from build123d import *

# Parameters (mm, degrees)
F1_DEPTH  = 16
F3_DEPTH  = 25
F4_SIZE   = 1
F11_ANGLE = 180
F14_DEPTH = 2
F16_DEPTH = 2


with BuildPart() as f1:
    # F0 (on Right) → F1 (new body)
    with BuildSketch(Plane.YZ):
        with BuildLine():
            Line((0, 7), (0, 0))
            Line((0, 0), (150, 0))
            Line((150, 0), (150, 7))
            ThreePointArc((150, 7), (148.5355339059, 10.5355339059), (145, 12))
            Line((145, 12), (128.050036002, 10.517070303))
            Line((128.050036002, 10.517070303), (127.1432693018, 20.8814611121))
            Line((127.1432693018, 20.8814611121), (113.1965435286, 19.6612807136))
            Line((113.1965435286, 19.6612807136), (113.8937894705, 11.6917231289))
            Line((113.8937894705, 11.6917231289), (5.5800139851, 2.2154956702))
            Line((5.5800139851, 2.2154956702), (4.9427024368, 9.5))
            Line((4.9427024368, 9.5), (20, 9.5))
            Line((20, 9.5), (20, 12))
            Line((20, 12), (5, 12))
            ThreePointArc((5, 12), (1.4644660941, 10.5355339059), (0, 7))
        make_face()
    extrude(amount=F1_DEPTH)

    # F2 (on face) → F3 (cut)
    with BuildSketch(Plane(origin=(0, 114.0437613881, 9.9775362673), x_dir=(1, 0, 0), z_dir=(0, -0.9961946981, -0.0871557427))):
        with BuildLine():
            Line((6, 9.7207347769), (6, 6.8026639789))
            ThreePointArc((6, 6.8026639789), (8, 2.6707347769), (10, 6.8026639789))
            Line((10, 6.8026639789), (10, 9.7207347769))
            Line((10, 9.7207347769), (11.5, 9.7207347769))
            ThreePointArc((11.5, 9.7207347769), (12.2071067812, 9.4278415581), (12.5, 8.7207347769))
            Line((12.5, 8.7207347769), (12.5, 4.7207347769))
            ThreePointArc((12.5, 4.7207347769), (13.3786796564, 2.5994144334), (15.5, 1.7207347769))
            Line((15.5, 1.7207347769), (18.5, 1.7207347769))
            Line((18.5, 1.7207347769), (18.5, 10.7207347769))
            Line((18.5, 10.7207347769), (-2.5, 10.7207347769))
            Line((-2.5, 10.7207347769), (-2.5, 1.7207347769))
            Line((-2.5, 1.7207347769), (0.5, 1.7207347769))
            ThreePointArc((0.5, 1.7207347769), (2.6213203436, 2.5994144334), (3.5, 4.7207347769))
            Line((3.5, 4.7207347769), (3.5, 8.7207347769))
            ThreePointArc((3.5, 8.7207347769), (3.7928932188, 9.4278415581), (4.5, 9.7207347769))
            Line((4.5, 9.7207347769), (6, 9.7207347769))
        make_face()
    extrude(amount=-F3_DEPTH, mode=Mode.SUBTRACT)

    # F4
    f4_edges = [f1.edges().sort_by_distance(p)[0] for p in [
        (6, 120.169906, 20.271371),
        (10, 120.169906, 20.271371),
    ]]
    chamfer(f4_edges, length=F4_SIZE)


with BuildPart() as f5_1:
    # F5: copy of F1
    add(f1.part.moved(Location((30, 0, 0))))


with BuildPart() as f6_1:
    # F6: copy of F5_1
    add(f5_1.part.moved(Location((30, 0, 0))))


with BuildPart() as f7_1:
    # F7: copy of F1
    add(f1.part.moved(Location((0, 160, 0))))


with BuildPart() as f8_1:
    # F8: copy of F5_1
    add(f5_1.part.moved(Location((0, 160, 0))))


with BuildPart() as f9_1:
    # F9: copy of F6_1
    add(f6_1.part.moved(Location((0, 160, 0))))


with BuildPart() as f8_1_1:
    # F11: moved
    add(f8_1.part.rotate(Axis((0, 0, 25), (0, 0, 1)), F11_ANGLE))


with BuildPart() as f9_1_1:
    # F11: moved
    add(f9_1.part.rotate(Axis((0, 0, 25), (0, 0, 1)), F11_ANGLE))


with BuildPart() as f7_1_1:
    # F11: moved
    add(f7_1.part.rotate(Axis((0, 0, 25), (0, 0, 1)), F11_ANGLE))


with BuildPart() as f7_1_2:
    # F12: moved
    add(f7_1_1.part.moved(Location((91, 310, 0))))

    # F13 (on face) → F14 (join)
    with BuildSketch(Plane.YZ.offset(91)):
        with BuildLine():
            Line((0, 7), (0, 0))
            Line((0, 0), (150, 0))
            Line((150, 0), (150, 7))
            ThreePointArc((150, 7), (148.5355339059, 10.5355339059), (145, 12))
            Line((145, 12), (5, 12))
            ThreePointArc((5, 12), (1.4644660941, 10.5355339059), (0, 7))
        make_face()
    extrude(amount=F14_DEPTH)


with BuildPart() as f8_1_2:
    # F12: moved
    add(f8_1_1.part.moved(Location((91, 310, 0))))


with BuildPart() as f9_1_2:
    # F12: moved
    add(f9_1_1.part.moved(Location((91, 310, 0))))


with BuildPart() as f1_1:
    add(f1.part)

    add(f5_1.part)  # F16 merges F5_1

    add(f6_1.part)  # F16 merges F6_1

    add(f7_1_2.part)  # F16 merges F7_1

    add(f8_1_2.part)  # F16 merges F8_1

    add(f9_1_2.part)  # F16 merges F9_1
    # F15 (on face) → F16 (join)
    with BuildSketch(Plane(origin=(0, 0, 0), x_dir=(0, -1, 0), z_dir=(-1, 0, 0))):
        with BuildLine():
            Line((-150, 0), (0, 0))
            Line((0, 0), (0, 7))
            ThreePointArc((0, 7), (-1.4644660941, 10.5355339059), (-5, 12))
            Line((-5, 12), (-145, 12))
            ThreePointArc((-145, 12), (-148.5355339059, 10.5355339059), (-150, 7))
            Line((-150, 7), (-150, 0))
        make_face()
    extrude(amount=F16_DEPTH)


solid = f1_1.part
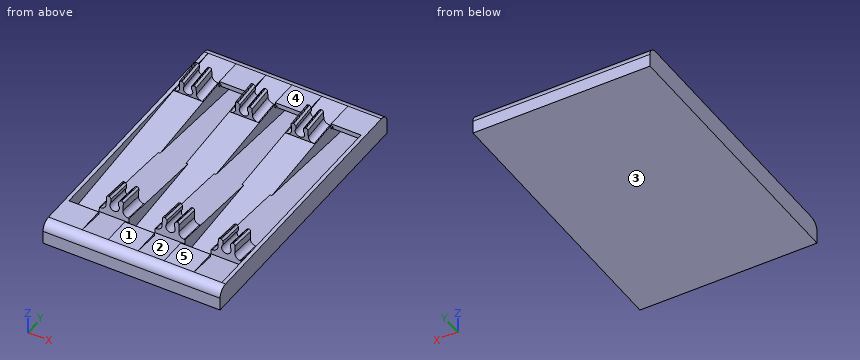
Source: CAD feature listing. Evaluate the final solid. Frame: model axes, mm. Face numbers are marked on the shaded views. A direction names the side the tool comes from. Give positions to 0.01 mm unless a question says otherwise; leave off trailing zeros. Order: outer loops, then holes, each group sorted by start corner. A loop starts at its lowest first (then second) coordinate and runs counter-clockwise, first axis right, second up. Notation, with made-up numbers: (83, 55) -> (136, 55) arc R24 ccw to (136, 75) -> close; hole circle Ø8 at (2, 39.25). An arc over 180 degrees is marked (long way). Write item = value, one per line.
Q1. Set-up query: the marked faces 3, 4 and 5. Return all of +Z, -Z, +X, -X, +Y, -Y with unobstructed straight access to the full face (end or side cutting, diameter ignored); none if empty.
Data:
face_3 = -Z, +X, -X, +Y, -Y
face_4 = +Z, +X, -X, +Y
face_5 = +Z, +X, -X, -Y
Q2. Pull-direction query (Y, two-part tool) for the marked faces 1 and 2; classes: released by +Y, released by -Y, zero draft, split by the parting line, or undercut.
Data:
face_1 = zero draft
face_2 = undercut
Q3. Cut plane D-D, the plane y = 17. Output: boundary loops of the cut face in (x, z), and give its area (3 significant figures).
Data:
outline = (-2, 0) -> (93, 0) -> (93, 12) -> (91, 12) -> (91, 10.95) -> (76, 10.95) -> (76, 12) -> (60, 12) -> (60, 10.95) -> (46, 10.95) -> (46, 12) -> (30, 12) -> (30, 10.95) -> (16, 10.95) -> (16, 12) -> (-2, 12) -> close; hole (0, 3.21) -> (15, 3.21) -> (15, 9.5) -> (0, 9.5) -> close; hole (31, 3.21) -> (45, 3.21) -> (45, 9.5) -> (31, 9.5) -> close; hole (61, 3.21) -> (75, 3.21) -> (75, 9.5) -> (61, 9.5) -> close
area = 825 mm^2
Q4. Cut plane B-B, the plane y = 66.5. Output: boundary loops of the cut face in (x, z), and give its area (3 significant figures).
Data:
outline = (-2, 0) -> (93, 0) -> (93, 12) -> (91, 12) -> (91, 9.03) -> (75, 9.03) -> (75, 7.55) -> (61, 7.55) -> (61, 9.03) -> (45, 9.03) -> (45, 7.55) -> (31, 7.55) -> (31, 9.03) -> (15, 9.03) -> (15, 7.55) -> (0, 7.55) -> (0, 12) -> (-2, 12) -> close
area = 806 mm^2
Q5. Pin query (flat end, axial travel): pin 1 (1.6 mm diameter, centred on y = 28.5, z = 17.5, fed in from +X); pin 2 (2.5 mm diameter, centred on y = 123.5, z = 18, fed in from +X); pin 3 (2 mm diameter, centred on x = 12, z = 11, fed in from +Y). Return the tip coordinate at first contact, or that it passes through.
Data:
pin_1 = 87.5
pin_2 = 72.5
pin_3 = 149
Q6. Material intervals for line 1 (X direction, y = 114, z = 5.5); line 2 (X direction, y = 108.5, z = 11.75); line 3 (Z direction, x = 2, y = 44), sorted ascending. Write a range as from..to.
Data:
line_1 = -2..16, 30..46, 60..76, 91..93
line_2 = -2..0, 91..93
line_3 = 0..5.58
Q7. Cut plane A-A, the plane z = 5.5. Output: boundary loops of the cut face in (x, y).
Data:
outline = (-2, 0) -> (93, 0) -> (93, 150) -> (-2, 150) -> close; hole (0, 5.29) -> (15, 5.29) -> (15, 43.12) -> (0, 43.12) -> close; hole (16, 106.88) -> (30, 106.88) -> (30, 144.71) -> (16, 144.71) -> close; hole (31, 5.29) -> (45, 5.29) -> (45, 43.12) -> (31, 43.12) -> close; hole (46, 106.88) -> (60, 106.88) -> (60, 144.71) -> (46, 144.71) -> close; hole (61, 5.29) -> (75, 5.29) -> (75, 43.12) -> (61, 43.12) -> close; hole (76, 106.88) -> (91, 106.88) -> (91, 144.71) -> (76, 144.71) -> close
Q8. Cut plane C-C, the plane x = 82.5. Output: boundary loops of the cut face in (y, z).
Data:
outline = (0, 0) -> (150, 0) -> (150, 7) arc R5 ccw to (145, 12) -> (130, 12) -> (130, 9.5) -> (145.06, 9.5) -> (144.42, 2.22) -> (36.11, 11.69) -> (36.19, 12.69) -> (22.25, 13.91) -> (21.95, 10.52) -> (5, 12) arc R5 ccw to (0, 7) -> close
